from build123d import *

# Parameters (mm, degrees)
BOSS_EXTRUDE1_DEPTH = 82.5
SKETCH4_W           = 165
SKETCH4_H           = 90
CUT_EXTRUDE1_DEPTH  = 10
SKETCH6_W           = 150
SKETCH6_H           = 122.5
CUT_EXTRUDE2_DEPTH  = 154.968340902
SKETCH7_W           = 80
SKETCH7_H           = 40
CUT_EXTRUDE3_DEPTH  = 60
SKETCH8_W           = 150
SKETCH8_H           = 2
BOSS_EXTRUDE2_DEPTH = 57.5
SKETCH9_W           = 20
SKETCH9_H           = 10
CUT_EXTRUDE4_DEPTH  = 211.059515376
SKETCH10_R          = 2
CUT_EXTRUDE5_DEPTH  = 6
CHAMFER1_SIZE       = 5
FILLET1_R           = 5
BOSS_EXTRUDE3_DEPTH = 10
SKETCH17_W          = 165
SKETCH17_H          = 130
BOSS_EXTRUDE4_DEPTH = 3.5
SKETCH16_R          = 2
CUT_EXTRUDE6_DEPTH  = 4
SKETCH19_R          = 1.6
SKETCH19_W          = 60
SKETCH19_H          = 35
CUT_EXTRUDE7_DEPTH  = 10


with BuildPart() as part:
    # Sketch2 → Boss-Extrude1 (new, symmetric)
    with BuildSketch(Plane(origin=(0, 0, 0), x_dir=(0, 0, -1), z_dir=(1, 0, 0))):
        Polygon((0, 112.583302492), (65, 0), (0, 0), (-65, 0), (-65, 112.583302492), align=None)
    extrude(amount=BOSS_EXTRUDE1_DEPTH, both=True)

    # Sketch4 → Cut-Extrude1 (cut)
    with BuildSketch(Plane(origin=(0, 28.145825623, -48.75), x_dir=(-1, 0, 0), z_dir=(0, 0.5000000000000044, -0.8660254037844362))):
        with Locations((0, 32.5)):
            Rectangle(SKETCH4_W, SKETCH4_H)
    extrude(amount=-CUT_EXTRUDE1_DEPTH, mode=Mode.SUBTRACT)

    # Sketch6 → Cut-Extrude2 (cut, through all)
    with BuildSketch(Plane(origin=(0, 112.583302492, 0), x_dir=(1, 0, 0), z_dir=(0, 1, 0))):
        with Locations((0, 3.75)):
            Rectangle(SKETCH6_W, SKETCH6_H)
    extrude(amount=-CUT_EXTRUDE2_DEPTH, mode=Mode.SUBTRACT)

    # Sketch7 → Cut-Extrude3 (cut)
    with BuildSketch(Plane.XY.offset(65)):
        with Locations((0, 20)):
            Rectangle(SKETCH7_W, SKETCH7_H)
    extrude(amount=-CUT_EXTRUDE3_DEPTH, mode=Mode.SUBTRACT)

    # Sketch8 → Boss-Extrude2 (add)
    with BuildSketch(Plane(origin=(0, 0, 57.5), x_dir=(-1, 0, 0), z_dir=(0, 0, -1))):
        with Locations((0, 41)):
            Rectangle(SKETCH8_W, SKETCH8_H)
    extrude(amount=BOSS_EXTRUDE2_DEPTH)

    # Sketch9 → Cut-Extrude4 (cut, through all)
    with BuildSketch(Plane.ZY.offset(82.5)):
        with Locations((33.170135622, 52)):
            Rectangle(SKETCH9_W, SKETCH9_H)
    extrude(amount=-CUT_EXTRUDE4_DEPTH, mode=Mode.SUBTRACT)

    # Sketch10 → Cut-Extrude5 (cut)
    with BuildSketch(Plane(origin=(0, 28.145825623, -48.75), x_dir=(-1, 0, 0), z_dir=(0, 0.5000000000000038, -0.8660254037844366))):
        with Locations(Location((-78.5, 89.25545404, 0), (0, 0, 90))):
            Circle(SKETCH10_R)
        with Locations(Location((78.5, 89.25545404, 0), (0, 0, 90))):
            Circle(SKETCH10_R)
        with Locations(Location((78.5, -25.24454596, 0), (0, 0, 90))):
            Circle(SKETCH10_R)
        with Locations(Location((-78.5, -25.74454596, 0), (0, 0, 90))):
            Circle(SKETCH10_R)
    extrude(amount=-CUT_EXTRUDE5_DEPTH, mode=Mode.SUBTRACT)

    # Chamfer1
    chamfer1_edges = [part.edges().sort_by_distance(p)[0] for p in [
        (57.5, 40, 57.5),
        (-57.5, 40, 57.5),
        (75, 40, 28.75),
        (-75, 40, 28.75),
    ]]
    chamfer(chamfer1_edges, length=CHAMFER1_SIZE)

    # Fillet1
    fillet1_edges = [part.edges().sort_by_distance(p)[0] for p in [
        (-78.75, 90.262794416, -1.339745962),
        (78.75, 12.320508076, -46.339745962),
        (-78.75, 12.320508076, -46.339745962),
        (78.75, 90.262794416, -1.339745962),
    ]]
    fillet(fillet1_edges, radius=FILLET1_R)

    # Sketch12 → Boss-Extrude3 (add)
    with BuildSketch(Plane.XZ):
        Polygon((82.5, 65), (40, 65), (40, 57.5), (75, 57.5), (75, -65), (82.5, -65), align=None)
        Polygon((-75, 57.5), (-40, 57.5), (-40, 65), (-82.5, 65), (-82.5, -65), (-75, -65), align=None)
    extrude(amount=BOSS_EXTRUDE3_DEPTH)

    # Sketch17 → Boss-Extrude4 (add)
    with BuildSketch(Plane.XZ.offset(10)):
        Rectangle(SKETCH17_W, SKETCH17_H)
    extrude(amount=BOSS_EXTRUDE4_DEPTH)

    # Sketch16 → Cut-Extrude6 (cut)
    with BuildSketch(Plane.XZ.offset(13.5)):
        with Locations(Location((-65, 60, 0), (0, 0, 270))):
            Circle(SKETCH16_R)
        with Locations(Location((65, 60, 0), (0, 0, 270))):
            Circle(SKETCH16_R)
        with Locations(Location((65, -60, 0), (0, 0, 270))):
            Circle(SKETCH16_R)
        with Locations(Location((-65, -60, 0), (0, 0, 270))):
            Circle(SKETCH16_R)
    extrude(amount=-CUT_EXTRUDE6_DEPTH, mode=Mode.SUBTRACT)

    # Sketch19 → Cut-Extrude7 (cut)
    with BuildSketch(Plane.XZ.offset(13.5)):
        with Locations(Location((-8, 59, 0), (0, 0, 270))):
            Circle(SKETCH19_R)
        with Locations(Location((8, 59, 0), (0, 0, 270))):
            Circle(SKETCH19_R)
        Rectangle(SKETCH19_W, SKETCH19_H)
    extrude(amount=-CUT_EXTRUDE7_DEPTH, mode=Mode.SUBTRACT)


solid = part.part
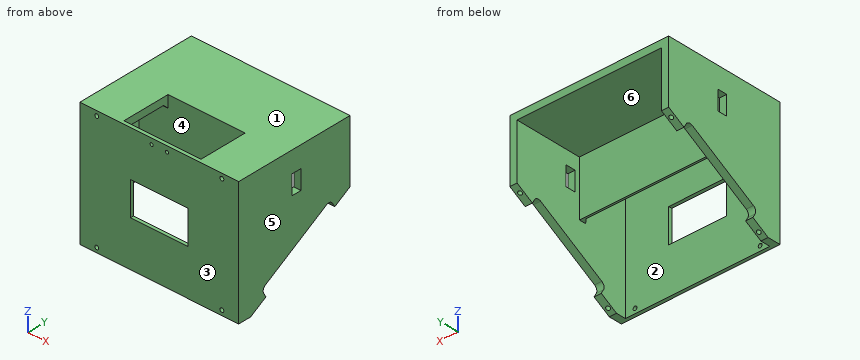
Here's how the part is built. I have some questions about the finished solid (model axes, mm). Face numbers are marked on the shaded views. A direction names the side the tool comes from. Coordinates: 2 decimals unless noted, no trailing zeros. Write each loop counter-clockwise with the first axis right and the second up, starting at its lowest first coordinate (ties: lowest second). Pieces come first, ordered by that corner, then holes. Notation, with made-up numbers: (-12.75, 79.25) - (15.25, 79.25) arc R16 ccw to (15.25, 90.25) - close; hole circle Ø1 at (-25, 72.25). An arc over 180 degrees is marked (long way). Use one line per item in the form item = value.
1) I'm going to push flat-ended pins straight in: P1, Ø5, axis at x = 65, z = -60, coming from the +Y side; P2, Ø8, axis at x = 24.5, y = 85.5, coming from the -Z side; P3, Ø2.5, axis at x = -65, z = -60, coming from the +Y side. Where does each tip first touch, or does it pass through?
Solved:
P1 = -10
P2 = 57.5
P3 = through
2) On a 3-axis mill with a long thin cutter (end or side, diameter ignored), from which of +Z, -Z, +X, -X, +Y, -Y can I reach the whole of each face in a straight line? I mean the marked faces 4, 5 and 6. Say none if no direction works.
Solved:
face_4 = -Z
face_5 = +Z, -Z, +X, +Y, -Y
face_6 = -Z, +Y
3) Suppose I cut it at B-B, the plane x = -32. Write out the boundary of the cut face in (y, z).
Solved:
outline = (-13.5, -65) - (-10, -65) - (-10, 65) - (-13.5, 65) - close; (40, 0) - (42, 0) - (42, 57.5) - (112.58, 57.5) - (112.58, 65) - (40, 65) - close
4) Suppose I cut it at D-D, the plane y = 29. Write out the boundary of the cut face in (x, z), plus the area to 3 significant figures.
Solved:
outline = (-82.5, -36.71) - (-75, -36.71) - (-75, 57.5) - (-40, 57.5) - (-40, 65) - (-82.5, 65) - close; (40, 57.5) - (75, 57.5) - (75, -36.71) - (82.5, -36.71) - (82.5, 65) - (40, 65) - close
area = 2,050 mm2
5) Thinking about a two-plate mould opening in Y: for the marked faces 1, 2 and 3, which applies, released by +Y, released by -Y, zero draft, split by the parting line, or undercut?
Solved:
face_1 = zero draft
face_2 = undercut
face_3 = released by -Y
6) I need wall thicknesses on line 1 (X direction, y = -12.55, z = -60); line 2 (Y direction, x = 67.5, z = 3); line 3 (X direction, y = 5.5, z = -5). Which ranges of each line are inside material? Lowest first, please.
Solved:
line_1 = -82.5 to -67, -63 to 63, 67 to 82.5
line_2 = -13.5 to -10, 40 to 42
line_3 = -82.5 to -75, 75 to 82.5
7) Suppose I cut it at A-A, the plane z = 40. Write out the boundary of the cut face in (x, y).
Solved:
outline = (-82.5, -13.5) - (82.5, -13.5) - (82.5, 47) - (75, 47) - (75, 42) - (-75, 42) - (-75, 47) - (-82.5, 47) - close; (-82.5, 57) - (-75, 57) - (-75, 112.58) - (-82.5, 112.58) - close; (75, 57) - (82.5, 57) - (82.5, 112.58) - (75, 112.58) - close; hole (-75, -10) - (75, -10) - (75, 35) - (70, 40) - (-70, 40) - (-75, 35) - close
8) Suppose I cut it at C-C, the plane x = -13. Write out the boundary of the cut face in (y, z).
Solved:
outline = (-13.5, -65) - (-10, -65) - (-10, -17.5) - (-13.5, -17.5) - close; (-13.5, 17.5) - (-10, 17.5) - (-10, 65) - (-13.5, 65) - close; (40, 0) - (42, 0) - (42, 57.5) - (112.58, 57.5) - (112.58, 65) - (40, 65) - close
